from build123d import *

# Parameters (mm, degrees)
SKETCH_2_W          = 0.1
SKETCH_2_H          = 3.5
CUT_EXTRUDE_1_DEPTH = 6


with BuildPart() as part:
    # 草图1 → 旋转1 (revolve)
    with BuildSketch(Plane.XY):
        Polygon((0.2, 3.5), (4.8, 3.5), (5, 3.427205953), (5, 2.6), (4.9, 2.5), (0.1, 2.5), (0, 2.6), (0, 3.427205953), align=None)
    revolve(axis=Axis((0, 0, 0), (1, 0, 0)))

    # 草图2 → 切除-拉伸1 (cut, through all)
    with BuildSketch(Plane(origin=(0, 0, 0), x_dir=(0, 0, -1), z_dir=(1, 0, 0))):
        with Locations((0, 1.75)):
            Rectangle(SKETCH_2_W, SKETCH_2_H)
    extrude(amount=CUT_EXTRUDE_1_DEPTH, mode=Mode.SUBTRACT)


solid = part.part
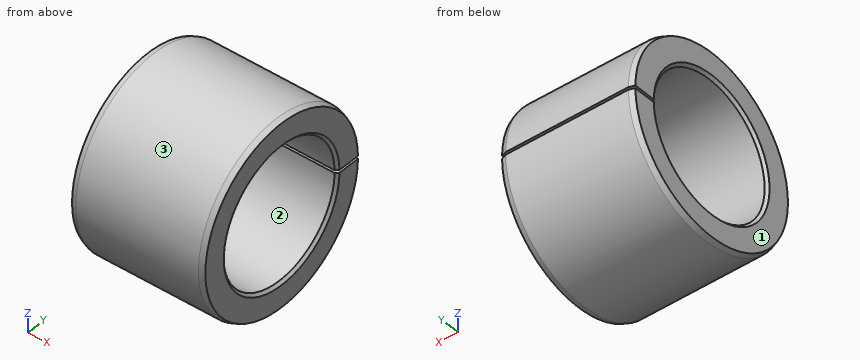
For this review, take the finished solid that the model builds, in its own axes (mm). Face numbers are marked on the shaded views. Give positions to 0.01 mm unless a question says otherwise; leave off trailing zeros. Order: outer loops, then holes, each group sorted by start corner. A loop starts at its lowest first (then second) coordinate and runs counter-clockwise, first axis right, second up. Notation, with made-up numbers: (58.25, 31.5) - (104.25, 31.5) arc R29 ccw to (104.25, 55.5) - close; hole circle Ø10 at (-5.75, 55). An arc over 180 degrees is marked (long way). Answer as a JSON object with one key per item and string values. Group by question number.
Item 1: Take a section at A-A on x = 1.15. Give the boundary of the cut face in (y, z), and give its area (3 significant figures).
Item 2: Draft analysis for pull direction Z (two halves, no side actions). For the marked faces 1, 2 and 3, state which applies: pulls with the +Z half, pulls with the -Z half, needs draft (parallel to the pull), parting line crosses it, or undercut.
Item 3: Wall thickness on line 1 along Z through (x, y) = (3.9, 0); line 2 along Y through (x, z) = (3.75, 0); line 3 along Z through (x, y) = (3.05, -2): over which ranges is each line inside the solid? List them lowest first.
Item 4: Clearance check with flat-ended pins moving along their axes: pin 1 Ø0.8 at (x, y) = (2.5, 3) entering from +Z; pin 2 Ø1.1 at (x, y) = (1.5, 3) entering from -Z; pin 3 Ø3 at (x, z) = (2, -2) entering from -Y. State where each tip first meets the part, or that it passes through.
Reported:
{
 "1": {"outline": "(2.5, -0.05) arc R2.5 cw (long way) to (2.5, 0.05) - (3.5, 0.05) arc R3.5 ccw (long way) to (3.5, -0.05) - close", "area": "18.7 mm^2"},
 "2": {"face 1": "needs draft", "face 2": "undercut", "face 3": "parting line crosses it"},
 "3": {"line 1": "-3.5 to -2.5, 2.5 to 3.5", "line 2": "-3.5 to -2.5", "line 3": "-2.87 to -1.5, 1.5 to 2.87"},
 "4": {"pin 1": "z = 2.34", "pin 2": "z = -2.5", "pin 3": "y = -3.46"}
}
